from build123d import *

# Parameters (mm, degrees)
BOSS_EXTRUDE1_DEPTH = 40.2
CUT_EXTRUDE1_START  = -3
CUT_EXTRUDE1_DEPTH  = 3
CUT_EXTRUDE4_DEPTH  = 40
SKETCH8_R           = 1.5
CUT_EXTRUDE5_DEPTH  = 40
FILLET2_R           = 2
SKETCH5_R           = 1.5
CUT_EXTRUDE6_DEPTH  = 73.958138682


# Read off the part's stored shape, not the designer's step: Cut-Extrude1
with BuildPart() as part:
    # Sketch1 → Boss-Extrude1 (new body)
    with BuildSketch(Plane.XY):
        with BuildLine():
            Line((-4.042288133, 0), (-42.7, 0))
            Line((-42.7, 0), (-42.7, 3))
            Line((-42.7, 3), (-3, 3))
            Line((-3, 3), (-3, 46.4))
            Line((-3, 46.4), (0, 46.4))
            Line((0, 46.4), (0, 3))
            ThreePointArc((0, 3), (-1.525340907, 0.831940258), (-4.042288133, 0))
        make_face()
    extrude(amount=BOSS_EXTRUDE1_DEPTH)

    # Cut-Extrude1 outline → Cut-Extrude1 (cut)
    with BuildSketch(Plane(origin=(0, 0, 0), x_dir=(0, 0, -1), z_dir=(1, 0, 0)).offset(CUT_EXTRUDE1_START)):
        with BuildLine():
            ThreePointArc((-40.2, 26.3), (-34.312846302, 40.512846302), (-20.1, 46.4))
            Line((-20.1, 46.4), (-40.2, 46.4))
            Line((-40.2, 46.4), (-40.2, 26.3))
        make_face()
        with BuildLine():
            ThreePointArc((-20.1, 46.4), (-5.887153698, 40.512846302), (0, 26.3))
            Line((0, 26.3), (0, 46.4))
            Line((0, 46.4), (-20.1, 46.4))
        make_face()
    extrude(amount=CUT_EXTRUDE1_DEPTH, mode=Mode.SUBTRACT)

    # Sketch7 → Cut-Extrude4 (cut)
    with BuildSketch(Plane(origin=(0, 0, 0), x_dir=(0, 0, -1), z_dir=(1, 0, 0))):
        with BuildLine():
            Line((-26.68, 34), (-26.68, 20))
            ThreePointArc((-26.68, 20), (-20.1, 13.42), (-13.52, 20))
            Line((-13.52, 20), (-13.52, 34))
            ThreePointArc((-13.52, 34), (-20.1, 40.58), (-26.68, 34))
        make_face()
    extrude(amount=-CUT_EXTRUDE4_DEPTH, mode=Mode.SUBTRACT)

    # Sketch8 → Cut-Extrude5 (cut)
    with BuildSketch(Plane(origin=(0, 0, 0), x_dir=(0, 0, -1), z_dir=(1, 0, 0))):
        with Locations(Location((-35.6, 27, 0), (0, 0, 90))):
            Circle(SKETCH8_R)
        with Locations(Location((-27.85, 40.423393759, 0), (0, 0, 90))):
            Circle(SKETCH8_R)
        with Locations(Location((-12.35, 40.423393759, 0), (0, 0, 90))):
            Circle(SKETCH8_R)
        with Locations(Location((-4.6, 27, 0), (0, 0, 90))):
            Circle(SKETCH8_R)
        with Locations(Location((-12.35, 13.576606241, 0), (0, 0, 90))):
            Circle(SKETCH8_R)
        with Locations(Location((-27.85, 13.576606241, 0), (0, 0, 90))):
            Circle(SKETCH8_R)
    extrude(amount=-CUT_EXTRUDE5_DEPTH, mode=Mode.SUBTRACT)

    # Fillet2
    fillet2_edges = [part.edges().sort_by_distance(p)[0] for p in [
        (-42.7, 1.5, 40.2),
        (-42.7, 1.5, 0),
    ]]
    fillet(fillet2_edges, radius=FILLET2_R)

    # Sketch5 → Cut-Extrude6 (cut, through all)
    with BuildSketch(Plane(origin=(0, 3, 0), x_dir=(1, 0, 0), z_dir=(0, 1, 0))):
        with Locations(Location((-10.5, -5, 0), (0, 0, 180))):
            Circle(SKETCH5_R)
        with Locations(Location((-10.5, -35.2, 0), (0, 0, 180))):
            Circle(SKETCH5_R)
        with Locations(Location((-34.7, -35.2, 0), (0, 0, 180))):
            Circle(SKETCH5_R)
        with Locations(Location((-34.7, -5, 0), (0, 0, 180))):
            Circle(SKETCH5_R)
    extrude(amount=-CUT_EXTRUDE6_DEPTH, mode=Mode.SUBTRACT)


solid = part.part
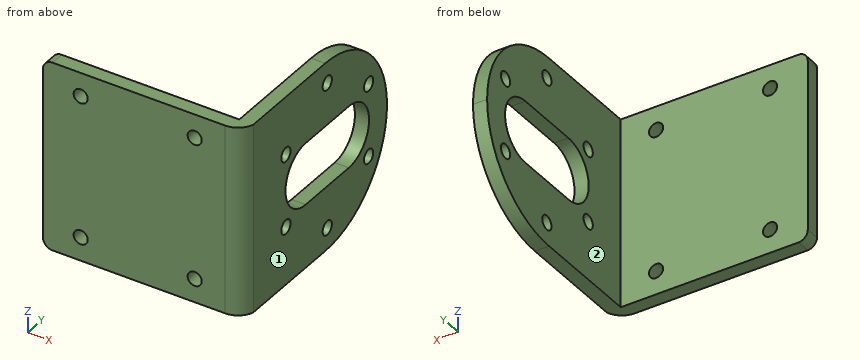
Geometry: final body of the model. Coordinates: model frame, mm. Face numbers are marked on the shaded views. A direction names the side the tool comes from. Round coordinates to 2 decimals unless told otherwise and drop trailing zeros. Loops run counter-clockwise (first coordinate to the right, second up) from the corner with the lowest first, then second, coordinate; pieces in that order, holes last.
Q1. Material intervals for L1, parallel to Z at x = -1.9, y = 27; L2, parallel to X at y = 41.5, z = 16; L3, parallel to Y at x = -23, z = 22.5, sorted ascending.
Q2. Pin query (flat end, axial travel): P1, Ø1.8, axis at y = 40.42, z = 27.85, coming from the -X side; P2, Ø2, axis at x = -28.5, z = 19, coming from the -Y side; P3, Ø5, axis at y = 33, z = 28.5, coming from the -X side; P4, Ø5, axis at x = -21.5, z = 6, coming from the +Y side. Return the tip coordinate at first contact, or that it passes through.
Q3. Section D-D on z = 18.5. Return loops of the section in (x, y).
Q4. Section B-B on z = 28.5. Return loops of the section in (x, y).
Q5. Access query for the marked faces 1 and 2. Directions: +Z, -Z, +X, -X, +Y, -Y. A direction counts if a zero-diameter tool reaches every point of the face in a straight line with its end or side. Return the directions, or none.
Q6. Section A-A on y = 27. Return loops of the section in (x, z).
Q7. Section C-C on y = 18. Return loops of the section in (x, z).
Evaluation:
1. L1: z = 0.01 to 3.1, 6.1 to 13.52, 26.68 to 34.1, 37.1 to 40.19
1. L2: x = -3 to 0
1. L3: y = 0 to 3
2. P1: passes through
2. P2: stops at y = 0
2. P3: stops at x = -3
2. P4: stops at y = 3
3. outline: (-42.7, 0) - (-4.04, 0) arc R4.22 ccw to (0, 3) - (0, 13.62) - (-3, 13.62) - (-3, 3) - (-42.7, 3) - close; (-3, 40.38) - (0, 40.38) - (0, 46.34) - (-3, 46.34) - close
4. outline: (-42.7, 0) - (-4.04, 0) arc R4.22 ccw to (0, 3) - (0, 12.22) - (-3, 12.22) - (-3, 3) - (-42.7, 3) - close; (-3, 14.93) - (0, 14.93) - (0, 39.07) - (-3, 39.07) - close; (-3, 41.78) - (0, 41.78) - (0, 44.56) - (-3, 44.56) - close
5. face 1: +Z, -Z, +X, +Y, -Y
5. face 2: +Z, -Z, -X, +Y
6. outline: (-3, 0.01) - (0, 0.01) - (0, 3.1) - (-3, 3.1) - close; (-3, 6.1) - (0, 6.1) - (0, 13.52) - (-3, 13.52) - close; (-3, 26.68) - (0, 26.68) - (0, 34.1) - (-3, 34.1) - close; (-3, 37.1) - (0, 37.1) - (0, 40.19) - (-3, 40.19) - close
7. outline: (-3, 0) - (0, 0) - (0, 13.83) - (-3, 13.83) - close; (-3, 26.37) - (0, 26.37) - (0, 40.2) - (-3, 40.2) - close
